Can you work these out from the drawing? Everything is in mm from the part's minimum corner. A direction names the side the tool comes from. Coordinates: 2 decimals unless noted, no trailing zeros. Order: outer loops, then holes, each group sorted by start corner. A loop starts at its lowest first (then second) coordinate and runs counter-clockwise, first axis right, second up. Notation, with made-up numbers: (17, -11) - (43, -11) arc R32 cw to (43, 20) - close; hole circle Ø2 at (-26.5, 70). An arc over 180 degrees is marked (long way). One line per item, written item: value.
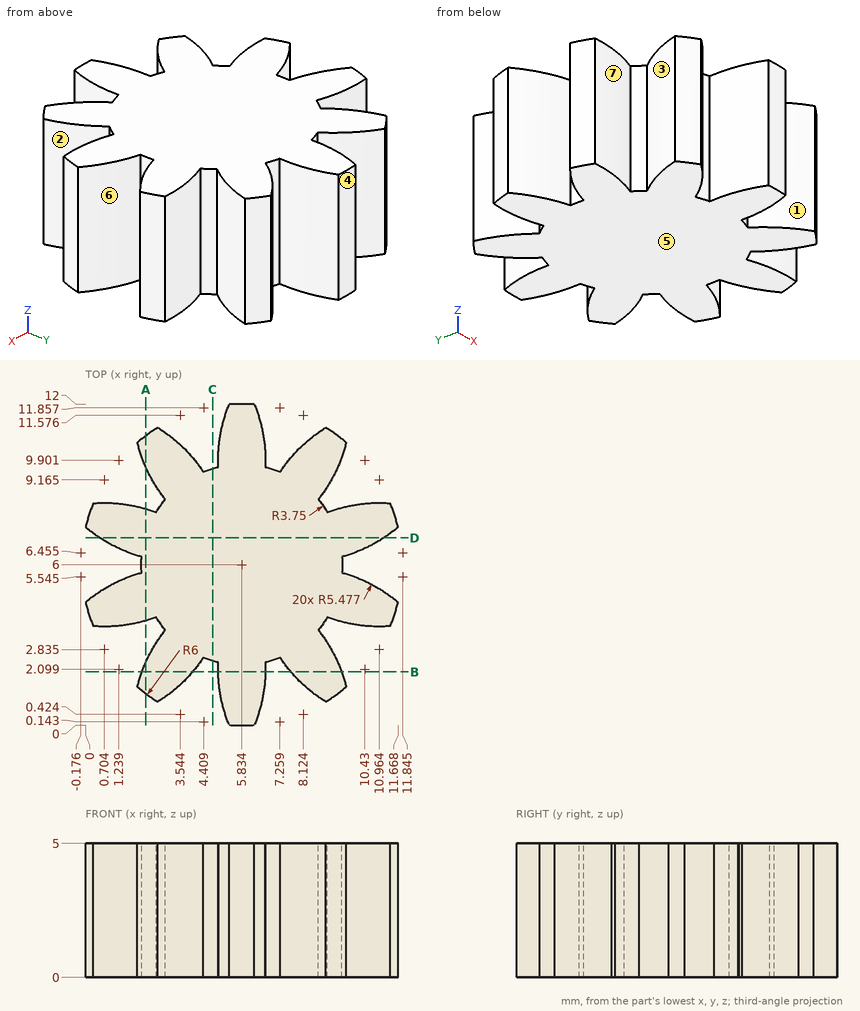
Item 1: I want a section at D-D on y = 7. Please give me the cut outline in (x, z) (1 decimal).
Conclusion:
outline: (0.5, 0) - (11.1, 0) - (11.1, 5) - (0.5, 5) - close
Item 2: I want a section at B-B on y = 2. Please give me the cut outline in (x, z) (1 decimal).
Conclusion:
outline: (2.1, 0) - (4, 0) - (4, 5) - (2.1, 5) - close; (5, 0) - (6.7, 0) - (6.7, 5) - (5, 5) - close; (7.7, 0) - (9.6, 0) - (9.6, 5) - (7.7, 5) - close
Item 3: Thinking about a two-plate mould opening in X: for the marked faces 4, 5, 6 and 7, which applies, pulls with the +X half, pulls with the -X half, needs draft (parallel to the pull), parting line crosses it, or undercut?
Conclusion:
face 4: parting line crosses it
face 5: needs draft
face 6: pulls with the +X half
face 7: undercut
Item 4: I want a section at A-A on x = 2.25. Please give me the cut outline in (y, z).
Conclusion:
outline: (1.19, 0) - (2.36, 0) - (2.36, 5) - (1.19, 5) - close; (3.91, 0) - (8.09, 0) - (8.09, 5) - (3.91, 5) - close; (9.64, 0) - (10.81, 0) - (10.81, 5) - (9.64, 5) - close
Item 5: I want a section at C-C on x = 4.75. Please give me the cut outline in (y, z), then the cut area to 3 significant figures.
Conclusion:
outline: (2.41, 0) - (9.59, 0) - (9.59, 5) - (2.41, 5) - close
area: 35.9 mm²
Item 6: For the marked faces 1, 2 and 3, which set-ups out of +Z, -Z, +X, -X, +Y, -Y let a thin tool reach every point of the face, with its end or its side?
Conclusion:
face 1: +Z, -Z, -Y
face 2: +Z, -Z, +X
face 3: +Z, -Z, -X
Item 7: I'm going to push flat-ended pins straight in: pin 1 Ø1.5 at (x, z) = (9.5, 4) entering from -Y; pin 2 Ø1 at (x, z) = (3.5, 4) entering from +Y (1 decimal); pin 3 Ø3 at (y, z) = (9.5, 2) entering from +X. Where does each tip first touch, or does it pass through?
Conclusion:
pin 1: y = 0.88
pin 2: y = 10.9
pin 3: x = 11.49
Item 8: If I drill on probe 1 along X at (y, z) = (9.75, 1.4) (1 decimal); probe 2 along Y at (x, z) = (10.25, 3.45) (1 decimal); probe 3 along X at (y, z) = (8.5, 3.9) (1 decimal), over which ranges is the centre line in solid material (lowest first)?
Conclusion:
probe 1: 2.2 to 4.2, 5 to 6.7, 7.5 to 9.5
probe 2: 3.7 to 5.5, 6.5 to 8.3
probe 3: 2.9 to 8.7
